```python
from build123d import *

# Parameters (mm, degrees)
F0_W     = 100
F0_H     = 120
F1_DEPTH = 6
F3_D     = 6.6
F4_R     = 8


with BuildPart() as f1:
    # F0 (on Front) → F1 (new body)
    with BuildSketch(Plane.XZ):
        with Locations((50, 60)):
            Rectangle(F0_W, F0_H)
    extrude(amount=F1_DEPTH)

    # F3 (through all)
    with Locations(Plane.XZ.offset(6)):
        with Locations((80, 30), (20, 40)):
            Hole(F3_D / 2)

    # F4
    f4_edges = [f1.edges().sort_by_distance(p)[0] for p in [
        (100, -3, 120),
        (100, -3, 0),
        (0, -3, 0),
        (0, -3, 120),
    ]]
    fillet(f4_edges, radius=F4_R)


solid = f1.part
```
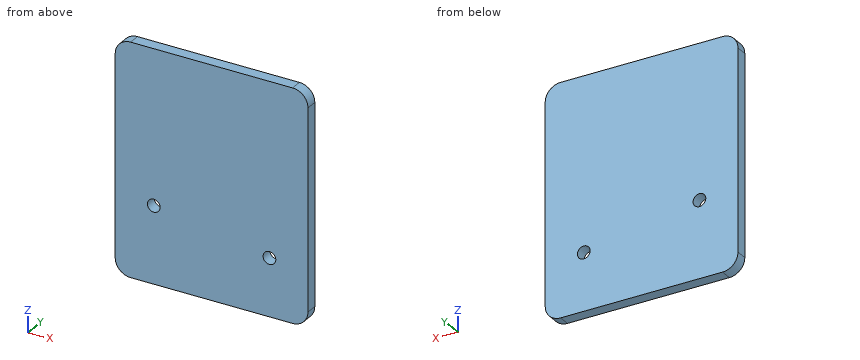
The model under review builds one solid part; all positions refer to its coordinate system, in mm. Round coordinates to 2 decimals unless told otherwise and drop trailing zeros. Write each loop counter-clockwise with the first axis right and the second up, starting at its lowest first coordinate (ties: lowest second). Pieces come first, ordered by that corner, then holes. Notation, with made-up numbers: (45.5, 51) - (78.5, 51) arc R23 ccw to (78.5, 72) - close; hole circle Ø11 at (7, 18). An arc over 180 degrees is marked (long way). Use one line per item in the form item = value.
Q1. Consider section B-B (x = 20). State the section outline as (y, z) points.
Answer key:
outline = (-6, 0) - (0, 0) - (0, 36.7) - (-6, 36.7) - close; (-6, 43.3) - (0, 43.3) - (0, 120) - (-6, 120) - close
Q2. For line 1 (Z direction, x = 20, y = -2.7); line 2 (Z direction, x = 80, y = -1.85), list the stretches that pass through material, from the lowest coordinate up. Write a range as [from, to].
Answer key:
line_1 = [0, 36.7], [43.3, 120]
line_2 = [0, 26.7], [33.3, 120]
Q3. Consider section A-A (z = 40). State the section outline as (x, y) points, and give its area (3 significant figures).
Answer key:
outline = (0, -6) - (16.7, -6) - (16.7, 0) - (0, 0) - close; (23.3, -6) - (100, -6) - (100, 0) - (23.3, 0) - close
area = 560 mm2
